```python
from build123d import *

# Parameters (mm, degrees)
SKETCH1_R           = 15
BOSS_EXTRUDE1_DEPTH = 2.5
SKETCH2_R           = 13.5
BOSS_EXTRUDE2_DEPTH = 0.5
SKETCH3_R           = 11.6
BOSS_EXTRUDE3_DEPTH = 5.3
SKETCH4_R           = 10.1
CUT_EXTRUDE1_DEPTH  = 5
CUT_EXTRUDE2_DEPTH  = 2
BOSS_EXTRUDE4_START = -2.5
BOSS_EXTRUDE4_DEPTH = 2.5
CUT_EXTRUDE3_DEPTH  = 1.5
CHAMFER1_SIZE       = 1.5
CHAMFER3_SIZE       = 1
CHAMFER3_SIZE_2     = 9.514364454


# Some blends are built 0.0001 mm under size
with BuildPart() as part:
    # Sketch1 → Boss-Extrude1 (new body)
    with BuildSketch(Plane(origin=(0, 0, 0), x_dir=(1, 0, 0), z_dir=(0, 1, 0))):
        with Locations(Location((0, 0, 0), (0, 0, 270))):
            Circle(SKETCH1_R)
    extrude(amount=BOSS_EXTRUDE1_DEPTH)

    # Sketch2 → Boss-Extrude2 (add)
    with BuildSketch(Plane(origin=(0, 2.5, 0), x_dir=(1, 0, 0), z_dir=(0, 1, 0))):
        with Locations(Location((0, 0, 0), (0, 0, 270))):
            Circle(SKETCH2_R)
    extrude(amount=BOSS_EXTRUDE2_DEPTH)

    # Sketch3 → Boss-Extrude3 (add)
    with BuildSketch(Plane(origin=(0, 3, 0), x_dir=(1, 0, 0), z_dir=(0, 1, 0))):
        with Locations(Location((0, 0, 0), (0, 0, 270))):
            Circle(SKETCH3_R)
    extrude(amount=BOSS_EXTRUDE3_DEPTH)

    # Sketch4 → Cut-Extrude1 (cut)
    with BuildSketch(Plane(origin=(0, 8.3, 0), x_dir=(1, 0, 0), z_dir=(0, 1, 0))):
        with Locations(Location((0, 0, 0), (0, 0, 270))):
            Circle(SKETCH4_R)
    extrude(amount=-CUT_EXTRUDE1_DEPTH, mode=Mode.SUBTRACT)

    # Sketch6 → Cut-Extrude2 (cut)
    with BuildSketch(Plane.XZ):
        with BuildLine():
            ThreePointArc((9.797958971, 2), (0, 10), (-9.797958971, 2))
            Line((-9.797958971, 2), (9.797958971, 2))
        make_face()
        with BuildLine():
            Line((9.797958971, -2), (-9.797958971, -2))
            ThreePointArc((-9.797958971, -2), (0, -10), (9.797958971, -2))
        make_face()
    extrude(amount=-CUT_EXTRUDE2_DEPTH, mode=Mode.SUBTRACT)

    # Sketch7 → Boss-Extrude4 (add)
    with BuildSketch(Plane(origin=(0, 8.3, 0), x_dir=(1, 0, 0), z_dir=(0, 1, 0)).offset(BOSS_EXTRUDE4_START)):
        with BuildLine():
            ThreePointArc((11.6, 0), (11.230512628, -2.904408047), (10.145588603, -5.623791595))
            Line((10.145588603, -5.623791595), (11.501249149, -6.375246506))
            ThreePointArc((11.501249149, -6.375246506), (12.731141471, -3.292497053), (13.15, 0))
            ThreePointArc((13.15, 0), (12.731141471, 3.292497053), (11.501249149, 6.375246506))
            Line((11.501249149, 6.375246506), (10.145588603, 5.623791595))
            ThreePointArc((10.145588603, 5.623791595), (11.230512628, 2.904408047), (11.6, 0))
        make_face()
        with BuildLine():
            Line((-11.501249149, -6.375246506), (-10.145588603, -5.623791595))
            ThreePointArc((-10.145588603, -5.623791595), (-11.6, 0), (-10.145588603, 5.623791595))
            Line((-10.145588603, 5.623791595), (-11.501249149, 6.375246506))
            ThreePointArc((-11.501249149, 6.375246506), (-13.15, 0), (-11.501249149, -6.375246506))
        make_face()
    extrude(amount=BOSS_EXTRUDE4_DEPTH)

    # Sketch8 → Cut-Extrude3 (cut)
    with BuildSketch(Plane.XZ):
        with BuildLine():
            Line((13, 3.5), (13, -3.5))
            Line((13, -3.5), (14.585952146, -3.5))
            ThreePointArc((14.585952146, -3.5), (14.896128393, -1.762202856), (15, 0))
            ThreePointArc((15, 0), (14.896128393, 1.762202856), (14.585952146, 3.5))
            Line((14.585952146, 3.5), (13, 3.5))
        make_face()
        with BuildLine():
            ThreePointArc((-14.585952146, 3.5), (-15, 0), (-14.585952146, -3.5))
            Line((-14.585952146, -3.5), (-13, -3.5))
            Line((-13, -3.5), (-13, 3.5))
            Line((-13, 3.5), (-14.585952146, 3.5))
        make_face()
    extrude(amount=-CUT_EXTRUDE3_DEPTH, mode=Mode.SUBTRACT)

    # Chamfer1
    chamfer1_edges = [part.edges().sort_by_distance(p)[0] for p in [
        (13, 1.5, 0),
        (-13, 1.5, 0),
    ]]
    chamfer(chamfer1_edges, length=CHAMFER1_SIZE - 0.0001)  # a hair under: the kernel refuses the full size

    # Chamfer3
    # the kernel refuses this chamfer: 9.514364454, 1 mm, written as the material it takes off along each edge
    with BuildSketch(Plane(origin=(33.132637154, 5.8, -18.365720673), x_dir=(-0.1658303097717397, 0.9396808679591152, -0.29916579809967064), z_dir=(-0.874619707139395, 0, 0.4848096202463386))) as chamfer3_piece_1_section:
        Polygon((CHAMFER3_SIZE * 0.939680867959, -CHAMFER3_SIZE * 0.342052432226), (-CHAMFER3_SIZE_2 * 0.342052432234, -CHAMFER3_SIZE_2 * 0.939680867981), (0, 0), align=None)
    chamfer3_piece_1 = extrude(amount=51.014670938, mode=Mode.PRIVATE)
    chamfer3_piece_1 = chamfer3_piece_1 - Plane(origin=(0, 6.124739453, 0), x_dir=(0, 0, 1), z_dir=(0, -1, 0)) * Cylinder(11.6, 138, mode=Mode.PRIVATE)
    add(chamfer3_piece_1, mode=Mode.SUBTRACT)
    with BuildSketch(Plane(origin=(-33.132637154, 5.8, 18.365720673), x_dir=(0.16583030977173743, 0.9396808679591152, 0.2991657980996716), z_dir=(0.8746197071393984, 0, -0.48480962024633234))) as chamfer3_piece_2_section:
        Polygon((CHAMFER3_SIZE * 0.939680867959, -CHAMFER3_SIZE * 0.342052432226), (-CHAMFER3_SIZE_2 * 0.342052432234, -CHAMFER3_SIZE_2 * 0.939680867981), (0, 0), align=None)
    chamfer3_piece_2 = extrude(amount=51.014670938, mode=Mode.PRIVATE)
    chamfer3_piece_2 = chamfer3_piece_2 - Plane(origin=(0, 6.124739453, 0), x_dir=(0, 0, 1), z_dir=(0, -1, 0)) * Cylinder(11.6, 138, mode=Mode.PRIVATE)
    add(chamfer3_piece_2, mode=Mode.SUBTRACT)


solid = part.part
```
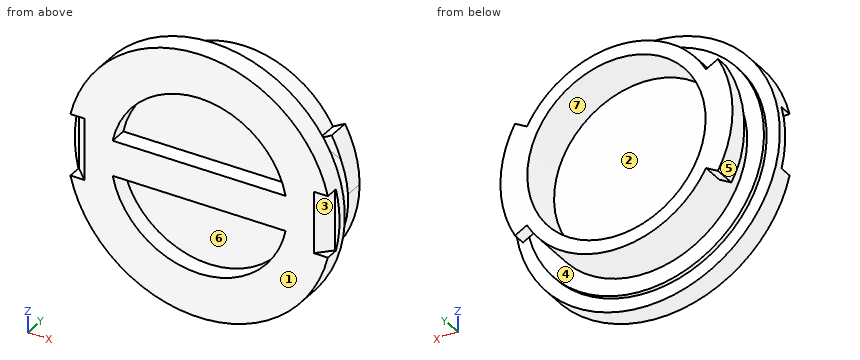
The listing builds one solid part. Answer for the finished solid, in the listing's coordinates (mm). Face numbers are marked on the shaded views. A direction names the side the tool comes from. Round coordinates to 2 decimals unless told otherwise and drop trailing zeros. Loops run counter-clockwise (first coordinate to the right, second up) from the corner with the lowest first, then second, coordinate; pieces in that order, holes last. Notation, with made-up numbers: (19.5, 73) -> (33.5, 73) arc R27 cw to (33.5, 94) -> close; hole circle Ø9 at (-11, -29). An arc over 180 degrees is marked (long way). Use one line per item in the form item = value.
1. The part is cut by section A-A on x = -12. Determine the outline of the cut face in (y, z).
Answer key:
outline = (0, -9) -> (2.5, -9) -> (2.5, -6.18) -> (3, -6.18) -> (3, 6.18) -> (2.5, 6.18) -> (2.5, 9) -> (0, 9) -> close; (5.8, -5.38) -> (8.3, -5.38) -> (8.3, 5.38) -> (6.68, 5.38) -> (5.8, -4.23) -> close
2. The part is cut by section B-B on x = 0. Determine the outline of the cut face in (y, z).
Answer key:
outline = (0, -15) -> (2.5, -15) -> (2.5, -13.5) -> (3, -13.5) -> (3, -11.6) -> (8.3, -11.6) -> (8.3, -10.1) -> (3.3, -10.1) -> (3.3, 10.1) -> (8.3, 10.1) -> (8.3, 11.6) -> (3, 11.6) -> (3, 13.5) -> (2.5, 13.5) -> (2.5, 15) -> (0, 15) -> (0, 10) -> (2, 10) -> (2, 2) -> (0, 2) -> (0, -2) -> (2, -2) -> (2, -10) -> (0, -10) -> close
3. A tool of negligible diameter and unlimited length cuts with its end or side. For the marked faces 4, 5, 6 and 7, from which of +Z, -Z, +X, -X, +Y, -Y can it reach the whole face along a straight path? Write none if from no direction.
Answer key:
face_4 = none
face_5 = -X, +Y
face_6 = -Y
face_7 = +Y
4. Find the intervals of material crossed by probe 1 along X at (y, z) = (6, 0); probe 2 along Y at (x, z) = (7, 13); probe 3 along X at (y, z) = (7.5, 8), in increasing order. Write a range as [from, to].
Answer key:
probe_1 = [-11.6, -10.1], [10.1, 11.6]
probe_2 = [0, 2.5]
probe_3 = [-8.4, -6.17], [6.17, 8.4]
5. The part is cut by section D-D on z = -12. Determine the outline of the cut face in (x, y), and give its area (3 significant figures).
Answer key:
outline = (-9, 0) -> (9, 0) -> (9, 2.5) -> (6.18, 2.5) -> (6.18, 3) -> (-6.18, 3) -> (-6.18, 2.5) -> (-9, 2.5) -> close
area = 51.2 mm²
6. The part is cut by section C-C on y = 4.25. Determine the outline of the cut face in (x, z).
Answer key:
outline = circle Ø23.2 at (0, 0); hole circle Ø20.2 at (0, 0)
7. Flat-ended cylindrical pins translate along their axes: pin 1 Ø2 at (x, z) = (0, 6) entering from +Y; pin 2 Ø1.5 at (y, z) = (4.5, -2) entering from -X; pin 3 Ø1.5 at (y, z) = (1, 5) entering from +X; pin 4 Ø2.5 at (x, z) = (11.5, 5.5) entering from -Y. Find the tip coordinate at first contact, or state that the pin passes through.
Answer key:
pin_1 = 3.3
pin_2 = -11.53
pin_3 = 14.39
pin_4 = 0
8. For a pull along X with two mould halves and no side action, classify the marked faces 1, 2 and 3 as released by +X, released by -X, zero draft, split by the parting line, or undercut.
Answer key:
face_1 = zero draft
face_2 = undercut
face_3 = released by +X
